from build123d import *

# Parameters (mm, degrees)
F0_W     = 1200
F0_H     = 600
F1_DEPTH = 25
F2_W     = 25
F2_H     = 600
F3_DEPTH = 675
F4_W     = 24.7376918793
F4_H     = 200
F4_W_2   = 26.8032312393
F5_DEPTH = 300
F6_W     = 24.7376918793
F6_H     = 200
F7_DEPTH = 25


with BuildPart() as f1:
    # F0 (on Top) → F1 (new body)
    with BuildSketch(Plane.XY):
        Rectangle(F0_W, F0_H)
    extrude(amount=F1_DEPTH)

    # F2 (on face) → F3 (join)
    with BuildSketch(Plane(origin=(0, 0, 0), x_dir=(1, 0, 0), z_dir=(0, 0, -1))):
        with Locations((-587.5, 0)):
            Rectangle(F2_W, F2_H)
        with Locations((587.5, 0)):
            Rectangle(F2_W, F2_H)
    extrude(amount=F3_DEPTH)

    # F4 (on face) → F5 (join)
    with BuildSketch(Plane.XY.offset(25)):
        with Locations((-587.6311540604, 200)):
            Rectangle(F4_W, F4_H)
        with Locations((586.5983843803, 200)):
            Rectangle(F4_W_2, F4_H)
    extrude(amount=F5_DEPTH)

    # F6 (on face) → F7 (join)
    with BuildSketch(Plane.XY.offset(325)):
        with Locations((-587.6311540604, 200)):
            Rectangle(F6_W, F6_H)
        Polygon((601.0820269585, 300), (-575.2623081207, 300), (-575.2623081207, 100), (-600, 100), (-600, 99.6639356017), (601.0820269585, 99.6639356017), align=None)
    extrude(amount=F7_DEPTH)


solid = f1.part
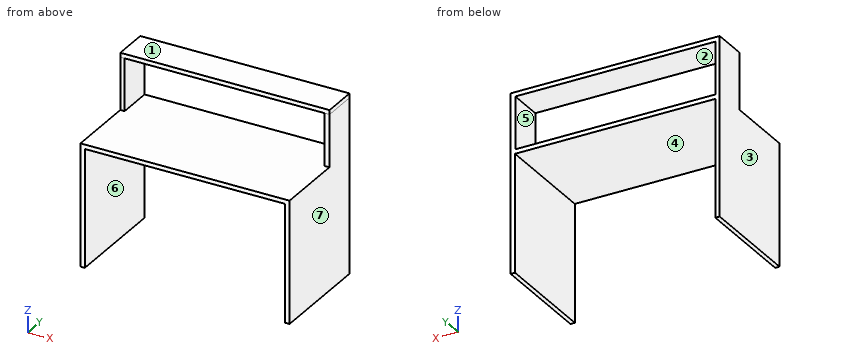
Input: part model. Units: mm. Frame: model coordinates. Face numbers are marked on the shaded views. A direction names the side the tool comes from. Give positions to 0.01 mm unless a question says otherwise; leave off trailing zeros. Write each loop counter-clockwise with the first axis right and the second up, starting at its lowest first coordinate (ties: lowest second). Pieces come first, ordered by that corner, then holes.
Q1. Set-up query: the marked faces 5, 6 and 7. Return all of +Z, -Z, +X, -X, +Y, -Y with unobstructed straight access to the full face (end or side cutting, diameter ignored); none if empty.
Q2. Material intervals for probe 1 along X at (y, z) = (81.5, -541.5); probe 2 along Z at (x, y) = (525, 106); probe 3 along Z at (x, y) = (48, 41), sorted ascending.
Q3. Section A-A, the plane z = -487.5. Output: boundary loops of the cut face in (x, y).
Q4. Section C-C, the plane y = 137. Output: boundary loops of the cut face in (x, z).
Q5. Section D-D, the plane y = -169.5. Output: boundary loops of the cut face in (x, z), plus the area to 4 significant figures.
Q6. Section B-B, the plane x = 63. Output: boundary loops of the cut face in (y, z), plus the area to 3 significant figures.
Q7. Pull-direction query (X, two-part tool) for the marked faces 1, 2, 3 and 4; classes: pulls with the +X half, pulls with the -X half, needs draft (parallel to the pull), parting line crosses it, or undercut.
Q8. First-contact query: P1, Ø12, axis at x = 163.5, y = 69, coming from the +Z side; P2, Ø10, axis at x = 46.5, y = 21, coming from the -Z side; P3, Ø10, axis at y = -236.5, z = -82, coming from the +X side. Flat tips, straight axial feed; report the tip coordinate or a pass-through.
Filled in:
1. face 5: +Y, -Y
1. face 6: -Z, +Y, -Y
1. face 7: -Z, +X, +Y, -Y
2. probe 1: x = -600 to -575, 575 to 600
2. probe 2: z = 0 to 25, 325 to 350
2. probe 3: z = 0 to 25
3. outline: (-600, -300) - (-575, -300) - (-575, 300) - (-600, 300) - close; (575, -300) - (600, -300) - (600, 300) - (575, 300) - close
4. outline: (-600, -675) - (-575, -675) - (-575, 0) - (575, 0) - (575, -675) - (600, -675) - (600, 325) - (601.08, 325) - (601.08, 350) - (-600, 350) - close; hole (-575.26, 25) - (573.2, 25) - (573.2, 325) - (-575.26, 325) - close
5. outline: (-600, -675) - (-575, -675) - (-575, 0) - (575, 0) - (575, -675) - (600, -675) - (600, 25) - (-600, 25) - close
5. area: 63,750 mm2
6. outline: (-300, 0) - (300, 0) - (300, 25) - (-300, 25) - close; (99.66, 325) - (300, 325) - (300, 350) - (99.66, 350) - close
6. area: 20,000 mm2
7. face 1: needs draft
7. face 2: undercut
7. face 3: pulls with the -X half
7. face 4: undercut
8. P1: stops at z = 25
8. P2: stops at z = 0
8. P3: stops at x = 600
